```python
from build123d import *

# Parameters (mm, degrees)
C_CHANNEL_120_X_12_5_DEPTH = 1870
SKETCH16_R                 = 3
CUT_EXTRUDE1_DEPTH         = 1876.299976004


with BuildPart() as part:
    # Sketch1 → C channel 120 X 12(5) (new body)
    with BuildSketch(Plane(origin=(0, 0, 0), x_dir=(-1, 0, 0), z_dir=(0, 1, 0))):
        with BuildLine():
            Line((65, 125), (0, 125))
            Line((0, 125), (0, 0))
            Line((0, 0), (65, 0))
            Line((65, 0), (65, 5.845330836))
            ThreePointArc((65, 5.845330836), (63.844151715, 8.856418565), (60.970378085, 10.320679365))
            Line((60.970378085, 10.320679365), (13.463772294, 15.313824837))
            ThreePointArc((13.463772294, 15.313824837), (8.354841396, 17.916955149), (6.3, 23.27))
            Line((6.3, 23.27), (6.3, 106.74))
            ThreePointArc((6.3, 106.74), (8.354841396, 112.093044851), (13.463772294, 114.696175163))
            Line((13.463772294, 114.696175163), (60.970378085, 119.689320635))
            ThreePointArc((60.970378085, 119.689320635), (63.844151715, 121.153581435), (65, 124.164669164))
            Line((65, 124.164669164), (65, 125))
        make_face()
    extrude(amount=C_CHANNEL_120_X_12_5_DEPTH)

    # Sketch16 → Cut-Extrude1 (cut, through all)
    with BuildSketch(Plane(origin=(0, 0, 0), x_dir=(0, 0, -1), z_dir=(1, 0, 0))):
        with Locations((-15.2, 280)):
            Circle(SKETCH16_R)
        with Locations((-15.2, 780)):
            Circle(SKETCH16_R)
        with Locations((-15.2, 1280)):
            Circle(SKETCH16_R)
        with Locations((-15.2, 1780)):
            Circle(SKETCH16_R)
    extrude(amount=-CUT_EXTRUDE1_DEPTH, mode=Mode.SUBTRACT)


solid = part.part
```
Verification items for the finished model (mm, model axes). A direction names the side the tool comes from. Round coordinates to 2 decimals unless told otherwise and drop trailing zeros. Order: outer loops, then holes, each group sorted by start corner. A loop starts at its lowest first (then second) coordinate and runs counter-clockwise, first axis right, second up. Notation, with made-up numbers: (5, 47) -> (47, 47) arc R23 ccw to (47, 61) -> close; hole circle Ø7 at (-24, -11). An arc over 180 degrees is marked (long way). Put each result on its own line as item: value. Start each with the question number.
(1) Section check B-B (z = 59). Enter the section's corners in (x, y).
(2) Tool access check on faces 4 (the face through (-33, 922, 125)), 5 (the face through (-36.885, 921.91, 117.158)). Record the directions out of +Z, -Z, +X, -X, +Y, -Y that give a thin tool (end or side, any length) a straight path to the whole face; none if there is none.
(3) Material ranges on line 1 along Y through (x, z) = (-13, 15); line 2 along Z through (x, y) = (-60.5, 1398.5); line 3 along Z through (x, y) = (-15, 270.5), recorded low to high.
(4) Section check A-A (y = 575). Enter the section's corners in (x, z), then the cut area to 3 significant figures.
(5) Depth check by flat-ended pin: pin 1 Ø6 at (x, y) = (-50.5, 780.5) entering from -Z; pin 2 Ø10 at (y, z) = (593.5, 50.5) entering from -X. Enter the tip coordinate at first touch or a pass-through.
(6) Draft check along Z on faces 1 (the face through (-6.3, 922, 64)), 2 (the face through (-6, 0, 54)), 3 (the face through (-32, 922, 0)). Enter one of: +Z half, -Z half, draft (parallel to the pull), parting line (faces both ways), or undercut.
Completed:
1. outline: (-6.3, 0) -> (0, 0) -> (0, 1870) -> (-6.3, 1870) -> close
2. face 4: +Z, +X, -X, +Y, -Y
2. face 5: -X, +Y, -Y
3. line 1: y = 0 to 277.01, 282.99 to 777.01, 782.99 to 1277.01, 1282.99 to 1777.01, 1782.99 to 1870
3. line 2: z = 0 to 10.37, 119.64 to 125
3. line 3: z = 0 to 15.15, 114.86 to 125
4. outline: (-65, 0) -> (0, 0) -> (0, 125) -> (-65, 125) -> (-65, 124.16) arc R4.5 ccw to (-60.97, 119.69) -> (-13.46, 114.7) arc R8 cw to (-6.3, 106.74) -> (-6.3, 23.27) arc R8 cw to (-13.46, 15.31) -> (-60.97, 10.32) arc R4.5 ccw to (-65, 5.85) -> close
4. area: 2,030 mm2
5. pin 1: stops at z = 0
5. pin 2: stops at x = -6.3
6. face 1: undercut
6. face 2: draft
6. face 3: -Z half
